Autodesk Inventor part; units mm, degrees
ref_plane "YZ Plane" through (0, 0, 0) normal (1, 0, 0) x (0, 1, 0)
ref_plane "XZ Plane" through (0, 0, 0) normal (0, 1, 0) x (-1, 0, 0)
ref_plane "XY Plane" through (0, 0, 0) normal (0, 0, 1) x (1, 0, 0)
sketch "Sketch1" plane through (0, 0, 0) normal (0, 1, 0) x (-1, 0, 0)
  line L0 (-15, 20) -> (15, 20)
  line L1 (15, 20) -> (15, -20)
  line L2 (15, -20) -> (-15, -20)
  line L3 (-15, -20) -> (-15, 20)
  line L4 (-15, 20) -> (15, -20) construction
  line L5 (15, 20) -> (-15, -20) construction
  point P0 (0, 0)
  dimension "d0" = 30
  dimension "d1" = 40
extrude "Extrusion1" add sketch "Sketch1" along normal blind 1
sketch "Sketch3" plane through (0, 1, 0) normal (0, 1, 0) x (1, 0, 0)
  line L0 (15, 20) -> (-15, 20)
  line L1 (-15, 20) -> (-2.4, 20)
  line L2 (-2.4, 20) -> (-2.4, 14)
  line L3 (-2.4, 14) -> (-15, 14)
  line L4 (-15, 14) -> (-15, 20)
  line L5 (0, 0) -> (0, 20) construction
  line L6 (15, 20) -> (2.4, 20)
  line L7 (2.4, 20) -> (2.4, 14)
  line L8 (2.4, 14) -> (15, 14)
  line L9 (15, 14) -> (15, 20)
  dimension "d7" = 12.6
  dimension "d8" = 6
  dimension "d9" = 12.6
  dimension "d10" = 6
extrude "Extrusion3" cut sketch "Sketch3" against normal up to surface (1 mm away)
sketch "Sketch8" plane through (0, 0, 0) normal (0, -1, 0) x (1, 0, 0)
  line L0 (2.4, -20) -> (-2.4, -20)
  line L1 (2.4, -20) -> (0, -20)
  line L2 (0, -20) -> (0, -17.5)
  line L3 (-2.4, -20) -> (-2.4, -14)
  line L4 (2.4, -20) -> (-2.4, -20)
  line L5 (-2.4, -20) -> (-2.4, -14)
  line L6 (-2.4, -14) -> (2.4, -14)
  line L7 (2.4, -14) -> (2.4, -20)
  line L8 (-15, 20) -> (15, 20)
  line L9 (15, 20) -> (10.15, 20)
  line L10 (15, 20) -> (19.85, 20) construction
  line L11 (10.15, 20) -> (10.15, 17.4)
  line L12 (10.15, 17.4) -> (-10.15, 17.4)
  line L13 (10.15, 17.4) -> (30.45, 17.4) construction
  circle A0 centre (-10.15, 17.4) radius 1.35
  circle A1 centre (10.15, 17.4) radius 1.35
  line L14 (15, 20) -> (15, -14)
  line L15 (15, 20) -> (-15, 20)
  line L16 (-15, 20) -> (-15, 15.5)
  line L17 (-15, 15.5) -> (15, 15.5)
  line L18 (15, 15.5) -> (15, 20)
  circle A2 centre (0, -17.5) radius 1.35
  point P0 (0, 0)
  dimension "d34" = 2.5
  dimension "d35" = 4.85
  dimension "d36" = 180
  dimension "d39" = 2.6
  dimension "d40" = 20.3
  dimension "d41" = 180
  dimension "d42" = 2.7
  dimension "d43" = 2.7
  dimension "d44" = 30
  dimension "d45" = 4.5
  dimension "d46" = 2.7
extrude "Extrusion7" add sketch "Sketch8" along normal blind 4.4
sketch "Sketch9" plane through (0, 0, 0) normal (0, -1, 0) x (1, 0, 0)
  circle A0 centre (10.15, 17.4) radius 1.35
  circle A1 centre (-10.15, 17.4) radius 1.35
  circle A2 centre (0, -17.5) radius 1.35
  point P0 (0, 0)
extrude "Extrusion8" cut sketch "Sketch9" against normal up to surface (1 mm away)
properties part number "imu_bottom_cover"
Can you work these out from the model? Positions are in its coordinate system, mm. A direction names the side the tool comes from. Coordinates: 2 decimals unless noted, no trailing zeros. Write each loop counter-clockwise with the first axis right and the second up, starting at its lowest first coordinate (ties: lowest second). Pieces come first, ordered by that corner, then holes. Notation, with made-up numbers: (7.25, 29) - (17.25, 29) arc R17 ccw to (17.25, 60) - close; hole circle Ø3 at (-25.5, 21). An arc over 180 degrees is marked (long way). Return JSON: item names as keys, results as strings. Group by question number.
Item 1: If we section it at C-C (z = -17.5): Write out the boundary of the cut face in (x, y), then the cut area to 3 significant figures.
Item 2: I'm going to push flat-ended pins straight in: pin 1 Ø1.6 at (y, z) = (-3, -17.5) entering from -X; pin 2 Ø2 at (x, y) = (-3.5, -1.5) entering from -Z; pin 3 Ø1.1 at (x, y) = (-9, 0.5) entering from -Z; pin 4 Ø1.6 at (x, z) = (0, -17.5) entering from +Y. Where does each tip first touch, or does it pass through?
Item 3: We'd pull the mould along X, two halves only. Please class faces 6 (the face through (15, 0.5, 8)), 7 (the face through (-1, -4.4, -16)), 8 (the face through (-10.44, -1.66, 18.72)): pulls with the +X half, pulls with the -X half, needs draft (parallel to the pull), parting line crosses it, or undercut.
Item 4: If we section it at B-B (x = 0): Write out the boundary of the cut face in (y, z), then the cut area to 3 significant figures.
Item 5: If we section it at D-D (y = 0.45): Write out the boundary of the cut face in (x, z).
Item 6: If we section it at A-A (y = -2.95): Write out the boundary of the cut face in (x, z).
Item 7: Which directions (+Z, -Z, +X, -X, +Y, -Y) give clear straight access to the entire face, cutting with the end or side of a thin tool? Please do faces 1 (the face through (-2.4, -2, -17)), 2 (the face through (0, -4.4, 18)), 3 (the face through (0, -2, -14)), 4 (the face through (0, -2, -20)), 5 (the face through (8.6, 0.5, -14)).
Item 8: Please list where these lines run through material, in increasing order: probe 1 along Z at (x, y) = (0, -2.05); probe 2 along Z at (x, y) = (-10.15, -0.4); probe 3 along Z at (x, y) = (1, 0.2).
Return value:
{
 "1": {"outline": "(-2.4, -4.4) - (-1.35, -4.4) - (-1.35, 1) - (-2.4, 1) - close; (1.35, -4.4) - (2.4, -4.4) - (2.4, 1) - (1.35, 1) - close", "area": "11.3 mm^2"},
 "2": {"pin 1": "stops at x = -2.4", "pin 2": "stops at z = 15.5", "pin 3": "stops at z = -14", "pin 4": "passes through"},
 "3": {"face 6": "pulls with the +X half", "face 7": "needs draft", "face 8": "undercut"},
 "4": {"outline": "(-4.4, -20) - (1, -20) - (1, -18.85) - (-4.4, -18.85) - close; (-4.4, -16.15) - (1, -16.15) - (1, 20) - (-4.4, 20) - (-4.4, 15.5) - (0, 15.5) - (0, -14) - (-4.4, -14) - close", "area": "71.6 mm^2"},
 "5": {"outline": "(-15, -14) - (-2.4, -14) - (-2.4, -20) - (2.4, -20) - (2.4, -14) - (15, -14) - (15, 20) - (-15, 20) - close; hole circle Ø2.7 at (-10.15, 17.4); hole circle Ø2.7 at (0, -17.5); hole circle Ø2.7 at (10.15, 17.4)"},
 "6": {"outline": "(-15, 15.5) - (15, 15.5) - (15, 20) - (-15, 20) - close; (-2.4, -20) - (2.4, -20) - (2.4, -14) - (-2.4, -14) - close; hole circle Ø2.7 at (-10.15, 17.4); hole circle Ø2.7 at (0, -17.5); hole circle Ø2.7 at (10.15, 17.4)"},
 "7": {"face 1": "-Z, -X, +Y, -Y", "face 2": "+Z, -Z, +X, -X, -Y", "face 3": "+X, -X, -Y", "face 4": "-Z, +X, -X, +Y, -Y", "face 5": "-Z, +X, +Y, -Y"},
 "8": {"probe 1": "z = -20 to -18.85, -16.15 to -14, 15.5 to 20", "probe 2": "z = 15.5 to 16.05, 18.75 to 20", "probe 3": "z = -20 to -18.41, -16.59 to 20"}
}
